Could you check a few things on this drawing? It's one solid part, dimensions in mm from its lowest x, y, z. Give positions to 0.01 mm unless a question says otherwise; leave off trailing zeros. Order: outer loops, then holes, each group sorted by start corner. A loop starts at its lowest first (then second) coordinate and runs counter-clockwise, first axis right, second up. Notation, with made-up numbers: (72, -21.5) -> (81, -21.5) arc R24 ccw to (81, 13.5) -> close; hole circle Ø11 at (68, 71.5). An arc over 180 degrees is marked (long way). Answer as a JSON object with one key per item and string values.
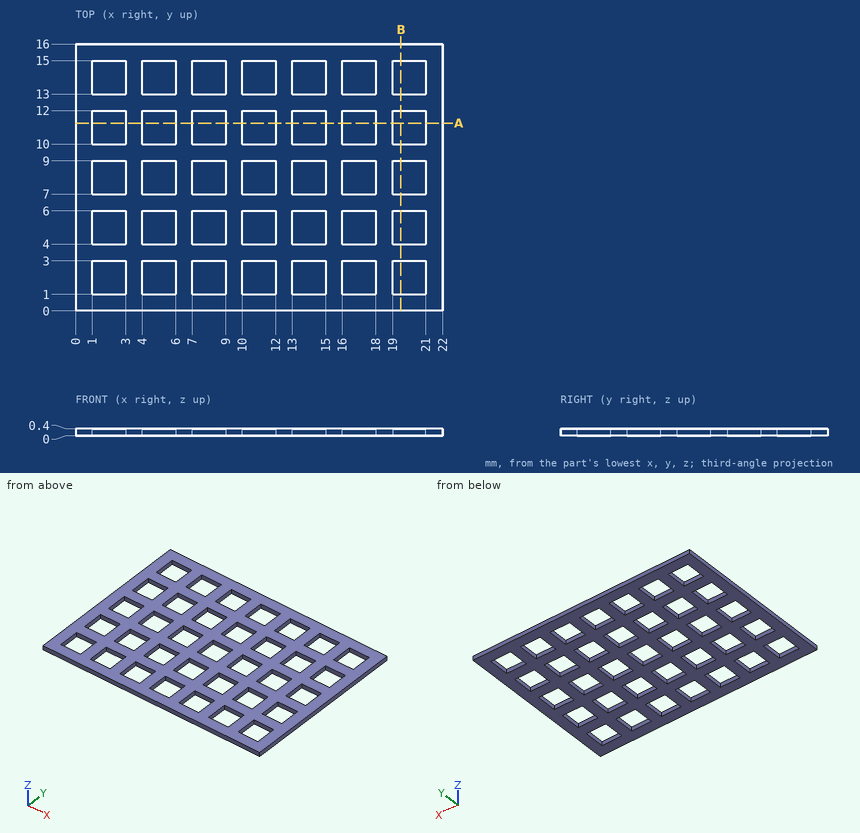
1. If we section it at A-A on y = 11.25: Count the separate pieces of the cut face and the enclosed holes in it, then the cut area to 3 significant figures.
Worked answers:
{"separate pieces": "8", "enclosed holes": "0", "area": "3.20 mm²"}
2. If we section it at B-B on x = 19.5: Please give me the cut outline in (y, z).
Worked answers:
{"outline": "(0, 0) -> (1, 0) -> (1, 0.4) -> (0, 0.4) -> close; (3, 0) -> (4, 0) -> (4, 0.4) -> (3, 0.4) -> close; (6, 0) -> (7, 0) -> (7, 0.4) -> (6, 0.4) -> close; (9, 0) -> (10, 0) -> (10, 0.4) -> (9, 0.4) -> close; (12, 0) -> (13, 0) -> (13, 0.4) -> (12, 0.4) -> close; (15, 0) -> (16, 0) -> (16, 0.4) -> (15, 0.4) -> close"}
3. Please list where this line runs through material, in increasing order: L1, parallel to Y at x = 8.75, z = 0.15.
Worked answers:
{"L1": "0 to 1, 3 to 4, 6 to 7, 9 to 10, 12 to 13, 15 to 16"}
